from build123d import *

# Parameters (mm, degrees)
EXTRUDE_1_DEPTH     = 5
EXTRUDE_5_DEPTH     = 5
CUT_EXTRUDE_2_REACH = 82.139
SKETCH_7_R          = 7.5
SKETCH_8_R          = 8.75
CUT_EXTRUDE_3_DEPTH = 1.3
CUT_EXTRUDE_4_REACH = 82.139
SKETCH_9_R          = 1.35
CUT_EXTRUDE_5_REACH = 82.139
SKETCH_12_R         = 2.1
SKETCH_14_W         = 40
SKETCH_14_H         = 7
EXTRUDE_6_DEPTH     = 15
CHAMFER_1_SIZE      = 7
CHAMFER_1_SIZE2     = 3
CUT_EXTRUDE_6_REACH = 134.447
SKETCH_15_R         = 2
FILLET_3_R          = 2
CHAMFER_2_SIZE      = 5
CUT_EXTRUDE_7_DEPTH = 15


with BuildPart() as part:
    # 草图1 → 凸台-拉伸1 (new body)
    with BuildSketch(Plane(origin=(0, 0, 0), x_dir=(1, 0, 0), z_dir=(0, 1, 0))):
        with BuildLine():
            Line((-65, 12.5), (65, 12.5))
            ThreePointArc((65, 12.5), (77.5, 0), (65, -12.5))
            Line((65, -12.5), (-65, -12.5))
            ThreePointArc((-65, -12.5), (-77.5, 0), (-65, 12.5))
        make_face()
    extrude(amount=EXTRUDE_1_DEPTH)

    # 草图10 → 凸台-拉伸5 (add)
    with BuildSketch(Plane.XZ):
        with BuildLine():
            Line((75.795454545, -6.301441197), (78.590909091, -1.512345887))
            ThreePointArc((78.590909091, -1.512345887), (79, 0), (78.590909091, 1.512345887))
            Line((78.590909091, 1.512345887), (75.795454545, 6.301441197))
            Line((75.795454545, 6.301441197), (75.795454545, -6.301441197))
        make_face()
    extrude(amount=-EXTRUDE_5_DEPTH)

    # 草图7 → 切除-拉伸2 (cut, up to next)
    with BuildSketch(Plane(origin=(0, 5, 0), x_dir=(1, 0, 0), z_dir=(0, 1, 0)), mode=Mode.PRIVATE) as cut_extrude_2_sk1:
        with Locations(Location((65, 0, 0), (0, 0, 270))):
            Circle(SKETCH_7_R)
    cut_extrude_2_tool1 = extrude(cut_extrude_2_sk1.sketch, amount=-CUT_EXTRUDE_2_REACH, mode=Mode.PRIVATE) & part.part
    add(cut_extrude_2_tool1.solids().sort_by_distance((65, 5, 0))[0], mode=Mode.SUBTRACT)

    # 草图8 → 切除-拉伸3 (cut)
    with BuildSketch(Plane(origin=(0, 0, 0), x_dir=(1, 0, 0), z_dir=(0, 1, 0))):
        with Locations(Location((65, 0, 0), (0, 0, 270))):
            Circle(SKETCH_8_R)
    extrude(amount=CUT_EXTRUDE_3_DEPTH, mode=Mode.SUBTRACT)

    # 草图9 → 切除-拉伸4 (cut, up to next)
    with BuildSketch(Plane.XZ, mode=Mode.PRIVATE) as cut_extrude_4_sk1:
        with Locations(Location((59.5, 9.526279442, 0), (0, 0, 270))):
            Circle(SKETCH_9_R)
    cut_extrude_4_tool1 = extrude(cut_extrude_4_sk1.sketch, amount=-CUT_EXTRUDE_4_REACH, mode=Mode.PRIVATE) & part.part
    # 草图9 → 切除-拉伸4 (cut, up to next)
    with BuildSketch(Plane.XZ, mode=Mode.PRIVATE) as cut_extrude_4_sk2:
        with Locations(Location((76, 0, 0), (0, 0, 270))):
            Circle(SKETCH_9_R)
    cut_extrude_4_tool2 = extrude(cut_extrude_4_sk2.sketch, amount=-CUT_EXTRUDE_4_REACH, mode=Mode.PRIVATE) & part.part
    # 草图9 → 切除-拉伸4 (cut, up to next)
    with BuildSketch(Plane.XZ, mode=Mode.PRIVATE) as cut_extrude_4_sk3:
        with Locations(Location((59.5, -9.526279442, 0), (0, 0, 270))):
            Circle(SKETCH_9_R)
    cut_extrude_4_tool3 = extrude(cut_extrude_4_sk3.sketch, amount=-CUT_EXTRUDE_4_REACH, mode=Mode.PRIVATE) & part.part
    add(cut_extrude_4_tool1.solids().sort_by_distance((59.5, 0, 9.526279))[0], mode=Mode.SUBTRACT)
    add(cut_extrude_4_tool2.solids().sort_by_distance((76, 0, 0))[0], mode=Mode.SUBTRACT)
    add(cut_extrude_4_tool3.solids().sort_by_distance((59.5, 0, -9.526279))[0], mode=Mode.SUBTRACT)

    # 草图12 → 切除-拉伸5 (cut, up to next)
    with BuildSketch(Plane(origin=(0, 5, 0), x_dir=(1, 0, 0), z_dir=(0, 1, 0)), mode=Mode.PRIVATE) as cut_extrude_5_sk1:
        with Locations(Location((-65, 0, 0), (0, 0, 270))):
            Circle(SKETCH_12_R)
    cut_extrude_5_tool1 = extrude(cut_extrude_5_sk1.sketch, amount=-CUT_EXTRUDE_5_REACH, mode=Mode.PRIVATE) & part.part
    add(cut_extrude_5_tool1.solids().sort_by_distance((-65, 5, 0))[0], mode=Mode.SUBTRACT)

    # 草图14 → 凸台-拉伸6 (add)
    with BuildSketch(Plane.XZ):
        with Locations((-32, -9)):
            Rectangle(SKETCH_14_W, SKETCH_14_H)
    extrude(amount=EXTRUDE_6_DEPTH)

    # 倒角1
    chamfer_1_edges = [part.edges().sort_by_distance(p)[0] for p in [
        (-52, -7.5, -5.5),
    ]]
    chamfer_1_side = [part.faces().sort_by_distance(p)[0] for p in [
        (-32, -7.5, -5.5),
    ]]
    chamfer(chamfer_1_edges, length=CHAMFER_1_SIZE, length2=CHAMFER_1_SIZE2, reference=chamfer_1_side[0])

    # 草图15 → 切除-拉伸6 (cut, up to next)
    with BuildSketch(Plane.ZY.offset(52), mode=Mode.PRIVATE) as cut_extrude_6_sk1:
        with Locations((-4.5, -12.5)):
            Circle(SKETCH_15_R)
    cut_extrude_6_tool1 = extrude(cut_extrude_6_sk1.sketch, amount=-CUT_EXTRUDE_6_REACH, mode=Mode.PRIVATE) & part.part
    add(cut_extrude_6_tool1.solids().sort_by_distance((-52, -12.5, -4.5))[0], mode=Mode.SUBTRACT)

    # 圆角3
    fillet_3_edges = [part.edges().sort_by_distance(p)[0] for p in [
        (-52, -7.5, -8.5),
        (-52, -7.5, -12.5),
        (-45, -14.616025404, -5.5),
        (-45, -5.383974596, -5.5),
        (-12, -5.383974596, -5.5),
        (-12, -7.5, -12.5),
    ]]
    fillet(fillet_3_edges, radius=FILLET_3_R - 0.0001)  # a hair under: the kernel refuses the full size

    # 倒角2
    chamfer_2_edges = [part.edges().sort_by_distance(p)[0] for p in [
        (-52, 0, -10.159413188),
        (-48.082601766, 0, -6.821115043),
        (-29.294702561, 0, -5.5),
        (-12, 0, -9),
        (-51.6696987, 0, -8.717799408),
        (-51.414242852, 0, -11.914242852),
        (-44.99161676, 0, -5.540842512),
        (-12.585757148, 0, -6.085757148),
        (-12.585757148, 0, -11.914242852),
    ]]
    chamfer(chamfer_2_edges, length=CHAMFER_2_SIZE)

    # 草图16 → 切除-拉伸7 (cut)
    with BuildSketch(Plane.XZ.offset(15)):
        Polygon((-61.333333333, -12.5), (-33.333333333, -0.5), (-61.333333333, -0.5), align=None)
    extrude(amount=-CUT_EXTRUDE_7_DEPTH, mode=Mode.SUBTRACT)


solid = part.part
Check sheet for the modelled part. Datum: model origin and axes. Units: mm. A direction names the side the tool comes from. Give positions to 0.01 mm unless a question says otherwise; leave off trailing zeros. Loops run counter-clockwise (first coordinate to the right, second up) from the corner with the lowest first, then second, coordinate; pieces in that order, holes last. Notation, with made-up numbers: M -33.75,-3 L -4.75,-3 A11 ccw -4.75,17 Z; hole C 38.5,64.25 d4. An arc over 180 degrees is marked long. Use a Markdown table: item, result. Add a question column.
Q1. Mould release check, pull along X, two halves, no side actions. Record for faces 4 (the flat face through (0, 5, 0)), 5 (the cylindrical face through (-66.863, 2.535, 0.969)), 6 (the flat face through (-10, -3, -9)), 7 (the conical face through (-52.77, -4.15, -9.16)): pulls with the +X half, pulls with the -X half, needs draft (parallel to the pull), parting line crosses it, or undercut.
Q2. Sectioned sample at A-A, the plane x = 59.5. Record the cut outline in (y, z).
Q3. Sectioned sample at B-B, the plane x = 1.5. Record the cut outline in (y, z).
Q4. Tool access check on faces 1 (the cylindrical face through (74.8, 2.46, -0.62)), 2 (the flat face through (-30, -8, -5.5)), 3 (the cylindrical face through (73.676, 0.641, -1.139)). Record the directions out of +Z, -Z, +X, -X, +Y, -Y that give a thin tool (end or side, any length) a straight path to the whole face; none if there is none.
Q5. Scan lines: line 1 along Z through (x, y) = (60, 3); line 2 along Y through (x, z) = (47, -3.25); line 3 along Z through (x, y) = (76, 1.9). Record each from-to range of solid material in increasing order. Write a range as [from, to].
Q6. Go/stop test with flat-tipped pins: pin 1 (12 mm diameter, centred on y = -7.5, z = -7, fed in from +X); pin 2 (2.5 mm diameter, centred on y = -10.5, z = -9.5, fed in from +X); pin 3 (6.5 mm diameter, centred on x = -26, y = -7, fed in from +Z). Record where each tip stops, or that it passes through.
Verdict:
| question | item | result |
|---|---|---|
| 1 | face 4 | needs draft |
| 1 | face 5 | undercut |
| 1 | face 6 | pulls with the +X half |
| 1 | face 7 | pulls with the -X half |
| 2 | outline | M 0,-12.5 L 5,-12.5 L 5,-10.88 L 0,-10.88 Z; M 0,-8.18 L 5,-8.18 L 5,-5.1 L 1.3,-5.1 L 1.3,-6.81 L 0,-6.81 Z; M 0,6.81 L 1.3,6.81 L 1.3,5.1 L 5,5.1 L 5,8.18 L 0,8.18 Z; M 0,10.88 L 5,10.88 L 5,12.5 L 0,12.5 Z |
| 3 | outline | M 0,-12.5 L 5,-12.5 L 5,12.5 L 0,12.5 Z |
| 4 | face 1 | +Y, -Y |
| 4 | face 2 | +Z, +X, -X, -Y |
| 4 | face 3 | -Y |
| 5 | line 1 | [-12.5, -10.78], [-8.27, -5.59], [5.59, 8.27], [10.78, 12.5] |
| 5 | line 2 | [0, 5] |
| 5 | line 3 | [-5.95, -1.35], [1.35, 5.95] |
| 6 | pin 1 | x = -8.51 |
| 6 | pin 2 | x = -12 |
| 6 | pin 3 | z = -4.25 |
